from build123d import *

# Parameters (mm, degrees)
ESQUISSE1_W             = 198
ESQUISSE1_H             = 106
ESQUISSE1_R             = 1.75
BOSS_EXTRU_1_DEPTH      = 3
ENL_V_MAT_EXTRU_1_DEPTH = 4


with BuildPart() as part:
    # Esquisse1 → Boss.-Extru.1 (new body)
    with BuildSketch(Plane.XY):
        Rectangle(ESQUISSE1_W, ESQUISSE1_H)
        with Locations((-86, -3)):
            Circle(ESQUISSE1_R, mode=Mode.SUBTRACT)
        with Locations((86, -3)):
            Circle(ESQUISSE1_R, mode=Mode.SUBTRACT)
    extrude(amount=BOSS_EXTRU_1_DEPTH)

    # Esquisse2 → Enlèv. mat.-Extru.1 (cut, through all)
    with BuildSketch(Plane(origin=(0, 0, 0), x_dir=(-1, 0, 0), z_dir=(0, 0, -1))):
        with BuildLine():
            Line((-15, 34), (15, 34))
            ThreePointArc((15, 34), (25, 24), (15, 14))
            Line((15, 14), (-15, 14))
            ThreePointArc((-15, 14), (-25, 24), (-15, 34))
        make_face()
    extrude(amount=-ENL_V_MAT_EXTRU_1_DEPTH, mode=Mode.SUBTRACT)


solid = part.part
Could you check a few things on this model? Use its own coordinates, in mm. A direction names the side the tool comes from. Give positions to 0.01 mm unless a question says otherwise; leave off trailing zeros. Write each loop counter-clockwise with the first axis right and the second up, starting at its lowest first coordinate (ties: lowest second). Pieces come first, ordered by that corner, then holes. Notation, with made-up numbers: (60, 25.25) - (92, 25.25) arc R21 cw to (92, 29.25) - close; hole circle Ø5 at (27, 24). An arc over 180 degrees is marked (long way). Use CSV: the item, a comma, the result in double quotes. Start each with the question number.
Item 1: I want a section at C-C, the plane y = 17. Please give me the cut outline in (x, z), then the cut area to 3 significant figures.
Item 2: If I drill on line 1 along Y through (x, z) = (86, 1.25); line 2 along Y through (x, z) = (14.5, 2.2); line 3 along X through (y, z) = (21, 0.9), over which ranges is the centre line in solid material (lowest first)?
Item 3: For faces 1 (the face through (25, 24, 1)), 2 (the face through (-1, 1, 3)), which set-ups out of +Z, -Z, +X, -X, +Y, -Y let a thin tool reach every point of the face, with its end or its side?
Item 4: I want a section at A-A, the plane x = -5. Please give me the cut outline in (y, z).
Item 5: I want a section at B-B, the plane z = 0.85. Please give me the cut outline in (x, y).
Item 6: If we mould it in two halves opening along X, with no side actions, what happens to faces 3 (the face through (-1, 1, 0)), 4 (the face through (87.669, -2.474, 1.479))? For each: pulls with the +X half, pulls with the -X half, needs draft (parallel to the pull), parting line crosses it, or undercut.
Findings:
1,outline,"(-99, 0) - (-22.14, 0) - (-22.14, 3) - (-99, 3) - close; (22.14, 0) - (99, 0) - (99, 3) - (22.14, 3) - close"
1,area,"461 mm2"
2,line 1,"y = -53 to -4.75, -1.25 to 53"
2,line 2,"y = -53 to 14, 34 to 53"
2,line 3,"x = -99 to -24.54, 24.54 to 99"
3,face 1,"+Z, -Z"
3,face 2,"+Z, +X, -X, +Y, -Y"
4,outline,"(-53, 0) - (14, 0) - (14, 3) - (-53, 3) - close; (34, 0) - (53, 0) - (53, 3) - (34, 3) - close"
5,outline,"(-99, -53) - (99, -53) - (99, 53) - (-99, 53) - close; hole circle Ø3.5 at (-86, -3); hole (-15, 14) - (15, 14) arc R10 ccw to (15, 34) - (-15, 34) arc R10 ccw to start; hole circle Ø3.5 at (86, -3)"
6,face 3,"needs draft"
6,face 4,"undercut"
